Verification items for the finished model (mm, model axes). Round coordinates to 2 decimals unless told otherwise and drop trailing zeros. Loops run counter-clockwise (first coordinate to the right, second up) from the corner with the lowest first, then second, coordinate; pieces in that order, holes last. Notation, with made-up numbers: M 73,26.25 L 132,26.25 A14 ccw 132,46.25 Z; hole C 68,-27.75 d6. An arc over 180 degrees is marked long. Write item = value, one per line. Start each with the question number.
from build123d import *

# Parameters (mm, degrees)
F1_DEPTH  = 5.842
F2_R      = 0.9525
F3_DEPTH  = 25.4
F5_W      = 0.889
F5_H      = 1.1938
F6_DEPTH  = 1.4097
F7_R      = 0.508
F9_DEPTH  = 1.8288
F11_DEPTH = 0.254
F12_W     = 1.016
F12_H     = 0.936952
F13_DEPTH = 25.4
F14_W     = 0.5842
F14_H     = 0.889
F15_DEPTH = 3.429


with BuildPart() as f1:
    # F0 (on Front) → F1 (new body)
    with BuildSketch(Plane.XZ):
        Polygon((0, 2.3368), (0, 0), (6.096, 0), (6.096, 12.8778), (0, 12.8778), (0, 10.5664), (-0.4572, 10.5664), (-0.4572, 8.2042), (0, 8.2042), (0, 4.7498), (-0.4572, 4.7498), (-0.4572, 2.3368), align=None)
    extrude(amount=F1_DEPTH)

    # F2 (on face) → F3 (cut)
    with BuildSketch(Plane.XZ.offset(5.842)):
        with Locations((1.076548, 9.7028)):
            Circle(F2_R)
        with Locations((1.076548, 3.2004)):
            Circle(F2_R)
    extrude(amount=-F3_DEPTH, mode=Mode.SUBTRACT)

    # F5 (on offset) → F6 (join, symmetric)
    with BuildSketch(Plane.XZ.offset(2.921)):
        with Locations((6.5405, 4.1021)):
            Rectangle(F5_W, F5_H)
    extrude(amount=F6_DEPTH, both=True)

    # F7
    f7_edges = [f1.edges().sort_by_distance(p)[0] for p in [
        (6.985, -2.921, 4.699),
        (6.985, -2.921, 3.5052),
    ]]
    fillet(f7_edges, radius=F7_R)

    # F8 (on offset) → F9 (join, symmetric)
    with BuildSketch(Plane.XZ.offset(2.921)):
        Polygon((6.096, 0.7112), (6.096, 0.4572), (6.477, 0.4572), (9.525, 13.699957), (9.277472, 13.756929), (6.274821, 0.7112), align=None)
    extrude(amount=F9_DEPTH, both=True)

    # F10 (on face) → F11 (cut)
    with BuildSketch(Plane(origin=(6.051205, 0, -1.392767), x_dir=(0, 1, 0), z_dir=(0.97452, 0, -0.224299))):
        Polygon((-4.7498, 9.518336), (-4.4831, 15.487336), (-4.7498, 15.487336), align=None)
        Polygon((-1.0922, 9.136269), (-1.0922, 15.487336), (-1.3589, 15.487336), align=None)
        with BuildLine():
            Line((-3.429, 9.010336), (-3.429, 1.898336))
            Line((-3.429, 1.898336), (-2.413, 1.898336))
            Line((-2.413, 1.898336), (-2.413, 9.010336))
            ThreePointArc((-2.413, 9.010336), (-2.56179, 9.369546), (-2.921, 9.518336))
            ThreePointArc((-2.921, 9.518336), (-3.28021, 9.369546), (-3.429, 9.010336))
        make_face()
    extrude(amount=-F11_DEPTH, mode=Mode.SUBTRACT)

    # F12 (on face) → F13 (cut)
    with BuildSketch(Plane.YZ.offset(6.096)):
        with Locations((-2.921, 0.633924)):
            Rectangle(F12_W, F12_H)
    extrude(amount=F13_DEPTH, mode=Mode.SUBTRACT)

    # F14 (on face) → F15 (join)
    with BuildSketch(Plane(origin=(0, 0, 0), x_dir=(0, -1, 0), z_dir=(-1, 0, 0))):
        with Locations((2.921, 6.3627)):
            Rectangle(F14_W, F14_H)
        with Locations((2.921, 11.4681)):
            Rectangle(F14_W, F14_H)
        with Locations((2.921, 1.2573)):
            Rectangle(F14_W, F14_H)
    extrude(amount=F15_DEPTH)


solid = f1.part
1. Section check D-D, the plane x = 5. Enter the section's corners in (y, z), and give its area (3 significant figures).
2. Section check A-A, the plane x = -2.5. Enter the section's corners in (y, z), and give its area (3 significant figures).
3. Thickness scan on line 1 (Z direction, x = -0.25, y = -3.45); line 2 (Z direction, x = 1.25, y = -1.5); line 3 (X direction, y = -4.2, z = 10.5). Record the ranges inside material, lowest first.
4. Section check C-C, the plane y = -3.65. Give the number of separate pieces and of enclosed holes in the cut face, and give its area (3 significant figures).
5. Mould release check, pull along Z, two halves, no side actions. Record for faces 1 (the flat face through (3, -3, 12.878)), 2 (the flat face through (-2, -3.213, 1)), 3 (the flat face through (7.8, -2.13, 7.33)), 4 (the cylindrical face through (0.37, -2.96, 3.84)): pulls with the +Z half, pulls with the -Z half, needs draft (parallel to the pull), parting line crosses it, or undercut.
6. Section check B-B, the plane z = 10. Enter the section's corners in (x, y), and give its area (3 significant figures).
7. Gauge pin test, flat ends, axial feed: P1, Ø3, axis at y = -3.5, z = 6, coming from the -X side; P2, Ø1, axis at x = -1.5, z = 11.5, coming from the +Y side; P3, Ø2, axis at y = -3, z = 7, coming from the +X side; P4, Ø0.6, axis at x = 7.5, z = 4, coming from the +Y side. Record the tip position at first contact, or that the pin passes through.
Computed values:
q1.outline = M -5.84,0 L 0,0 L 0,12.88 L -5.84,12.88 Z
q1.area = 75.2 mm2
q2.outline = M -3.21,0.81 L -2.63,0.81 L -2.63,1.7 L -3.21,1.7 Z; M -3.21,5.92 L -2.63,5.92 L -2.63,6.81 L -3.21,6.81 Z; M -3.21,11.02 L -2.63,11.02 L -2.63,11.91 L -3.21,11.91 Z
q2.area = 1.56 mm2
q3.line_1 = 2.34 to 4.75, 8.2 to 10.57
q3.line_2 = 0 to 2.26, 4.14 to 8.77, 10.64 to 12.88
q3.line_3 = -0.46 to 0.56, 1.6 to 6.1, 8.53 to 8.79
q4.separate_pieces = 1
q4.enclosed_holes = 2
q4.area = 79.4 mm2
q5.face_1 = pulls with the +Z half
q5.face_2 = needs draft
q5.face_3 = undercut
q5.face_4 = undercut
q6.outline = M -0.46,-5.84 L 0.17,-5.84 L 0.17,0 L -0.46,0 Z; M 1.98,-5.84 L 6.1,-5.84 L 6.1,0 L 1.98,0 Z; M 8.41,-4.66 L 8.67,-4.65 L 8.67,-1.2 L 8.41,-1.2 Z
q6.area = 28.6 mm2
q7.P1 = -3.43
q7.P2 = -2.63
q7.P3 = 8.21
q7.P4 = -1.09
